Here's how the part is built. I have some questions about the finished solid (model axes, mm). Face numbers are marked on the shaded views. A direction names the side the tool comes from. Give positions to 0.01 mm unless a question says otherwise; leave off trailing zeros. Write each loop counter-clockwise with the first axis right and the second up, starting at its lowest first coordinate (ties: lowest second). Pieces come first, ordered by that corner, then holes. Notation, with made-up numbers: M -32,-36 L -11,-36 A20 cw -11,-22 Z; hole C 81.5,-36.5 d5. An arc over 180 degrees is marked long. Answer as CSV lines item,"result". Start each with the question number.
Q1. Suppose I cut it at D-D (x = 0.25). Write out the boundary of the cut face in (y, z).
Q2. On a 3-axis mill with a long thin cutter (end or side, diameter ignored), from which of +Z, -Z, +X, -X, +Y, -Y can I reach the whole of each face in a straight line? I mean the marked faces 1 and 2. Say none if no direction works.
Q3. Suppose I cut it at C-C (x = 1.75). Write out the boundary of the cut face in (y, z).
Q4. For pin 1 (2 mm diameter, centred on x = 4, y = 5.5, fed in from +Z); pin 2 (3 mm diameter, centred on x = 5, z = 0, fed in from +Y), each with a flat end and sliding along its axis, tell me the tip position at first contact or that it passes through.
Q5. Suppose I cut it at A-A (y = 4.5). Write out the boundary of the cut face in (x, z).
Q6. Suppose I cut it at B-B (z = 3.25). Write out the boundary of the cut face in (x, y).
Q7. Thinking about a two-plate mould opening in Z: for the marked faces 3, 4 and 5, which applies, +Z half, -Z half, draft (parallel to the pull), parting line (faces both ways), or undercut?
Q8. If I drill on line 1 along Z through (x, y) = (2.5, 1.25); line 2 along Z through (x, y) = (0, 2.75); line 3 along Y through (x, z) = (0.25, 0.5), over which ranges is the centre line in solid material (lowest first)?
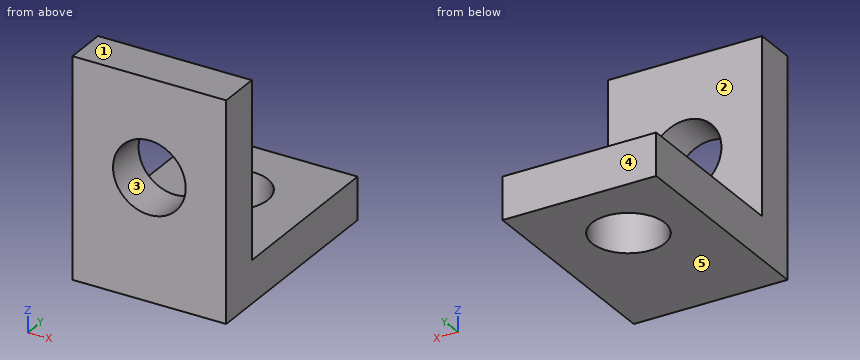
```python
from build123d import *

# Parameters (mm, degrees)
SKETCH1_W               = 6.35
SKETCH1_H               = 9
SKETCH1_R               = 1.5
BOSS_EXTRUDE1_DEPTH     = 1.75
SKETCH2_W               = 6.35
SKETCH2_H               = 1.75
BOSS_EXTRUDE2_DEPTH     = 7.25
SKETCH3_R               = 1.5
CUT_EXTRUDE1_DEPTH      = 8.25
CUT_EXTRUDE1_DEPTH_BACK = 2.75


with BuildPart() as part:
    # Sketch1 → Boss-Extrude1 (new body)
    with BuildSketch(Plane(origin=(0, 0, 0), x_dir=(1, 0, 0), z_dir=(0, 1, 0))):
        with Locations((2.570238095, -2.458928571)):
            Rectangle(SKETCH1_W, SKETCH1_H)
        with Locations((2.570238095, -2.958928571)):
            Circle(SKETCH1_R, mode=Mode.SUBTRACT)
    extrude(amount=BOSS_EXTRUDE1_DEPTH)

    # Sketch2 → Boss-Extrude2 (add)
    with BuildSketch(Plane(origin=(0, 1.75, 0), x_dir=(1, 0, 0), z_dir=(0, 1, 0))):
        with Locations((2.570238095, 1.166071429)):
            Rectangle(SKETCH2_W, SKETCH2_H)
    extrude(amount=BOSS_EXTRUDE2_DEPTH)

    # Sketch3 → Cut-Extrude1 (cut, two sides)
    with BuildSketch(Plane.XY.offset(-0.291071429)) as cut_extrude1_sk:
        with Locations((2.425238095, 5.875)):
            Circle(SKETCH3_R)
    extrude(amount=CUT_EXTRUDE1_DEPTH, mode=Mode.SUBTRACT)
    extrude(cut_extrude1_sk.sketch, amount=-CUT_EXTRUDE1_DEPTH_BACK, mode=Mode.SUBTRACT)


solid = part.part
```
Resolved:
1,outline,"M 0,-2.04 L 9,-2.04 L 9,-0.29 L 1.75,-0.29 L 1.75,6.96 L 0,6.96 Z"
2,face 1,"+Z, +X, -X, +Y, -Y"
2,face 2,"+Z, +X, -X, +Y"
3,outline,"M 0,-2.04 L 4.54,-2.04 L 4.54,-0.29 L 1.75,-0.29 L 1.75,1.7 L 0,1.7 Z; M 0,4.21 L 1.75,4.21 L 1.75,6.96 L 0,6.96 Z; M 7.21,-2.04 L 9,-2.04 L 9,-0.29 L 7.21,-0.29 Z"
4,pin 1,"z = -0.29"
4,pin 2,"y = 9"
5,outline,"M -0.6,-2.04 L 1.83,-2.04 L 1.83,-0.29 L -0.6,-0.29 Z; M 3.02,-2.04 L 5.75,-2.04 L 5.75,-0.29 L 3.02,-0.29 Z"
6,outline,"M -0.6,0 L 1.1,0 L 1.1,1.75 L -0.6,1.75 Z; M 4.04,0 L 5.75,0 L 5.75,1.75 L 4.04,1.75 Z"
7,face 3,"undercut"
7,face 4,"draft"
7,face 5,"-Z half"
8,line 1,"-2.04 to 1.46, 4.46 to 6.96"
8,line 2,"-2.04 to -0.29"
8,line 3,"0 to 1.75"
